Geometry check sheet. Reference: the model listing, model coordinates, mm. A direction names the side the tool comes from. Round coordinates to 2 decimals unless told otherwise and drop trailing zeros. One line per question, with ' | ' between items. Start each with the question number.
Q1. Gauge pin test, flat ends, axial feed: P1, Ø2.5, axis at y = 18.5, z = 26, coming from the -X side; P2, Ø3, axis at y = 230.5, z = 23.5, coming from the -X side; P3, Ø3, axis at y = 209.5, z = 26.5, coming from the -X side. Record the tip position at first contact, or that the pin passes through.
Q2. Tool access check on faces 1 (the face through (50, 20, 20)), 2 (the face through (-1, 15, 30)), 3 (the face through (-50, 21, 20)), 4 (the face through (59.14, 247.75, 37.97)). Record the directions out of +Z, -Z, +X, -X, +Y, -Y that give a thin tool (end or side, any length) a straight path to the whole face; none if there is none.
Q3. Material ranges on line 1 along X through (y, z) = (20, 23); line 2 along X through (y, z) = (155, 37); line 3 along X through (y, z) = (35, 16), recorded low to high.
Q4. Mould release check, pull along Y, two halves, no side actions. Record for faces 5 (the face through (4.78, 279.91, 19.76)), 6 (the face through (2, 157, 36)), 7 (the face through (40, 15, 20)): +Y half, -Y half, draft (parallel to the pull), parting line (faces both ways), or undercut.
```python
from build123d import *

# Parameters (mm, degrees)
SKETCH2_R           = 110
BOSS_EXTRUDE1_DEPTH = 40
SKETCH5_R           = 110
BOSS_EXTRUDE2_DEPTH = 36
FILLET1_R           = 3
SKETCH6_W           = 80
SKETCH6_H           = 20
CUT_EXTRUDE2_DEPTH  = 30
SKETCH7_W           = 70
SKETCH7_H           = 10
BOSS_EXTRUDE3_DEPTH = 30
SKETCH8_W           = 5
SKETCH8_H           = 30
BOSS_EXTRUDE4_DEPTH = 3


with BuildPart() as part:
    # Sketch2 → Boss-Extrude1 (new body)
    with BuildSketch(Plane.XY):
        with BuildLine():
            Line((-50, 0), (50, 0))
            Line((50, 0), (50, 40.435607626))
            ThreePointArc((50, 40.435607626), (0, 280), (-50, 40.435607626))
            Line((-50, 40.435607626), (-50, 0))
        make_face()
        with Locations((0, 155)):
            Circle(SKETCH2_R, mode=Mode.SUBTRACT)
    extrude(amount=BOSS_EXTRUDE1_DEPTH)

    # Sketch5 → Boss-Extrude2 (add)
    with BuildSketch(Plane(origin=(0, 0, 0), x_dir=(-1, 0, 0), z_dir=(0, 0, -1))):
        with Locations((0, 155)):
            Circle(SKETCH5_R)
    extrude(amount=-BOSS_EXTRUDE2_DEPTH)

    # Fillet1
    fillet1_edges = [part.edges().sort_by_distance(p)[0] for p in [
        (-50, 20.217803813, 40),
        (50, 20.217803813, 40),
        (-50, 20.217803813, 0),
        (0, 280, 0),
        (50, 20.217803813, 0),
        (0, 280, 40),
    ]]
    fillet(fillet1_edges, radius=FILLET1_R)

    # Sketch6 → Cut-Extrude2 (cut)
    with BuildSketch(Plane.XZ):
        with Locations((0, 20)):
            Rectangle(SKETCH6_W, SKETCH6_H)
    extrude(amount=-CUT_EXTRUDE2_DEPTH, mode=Mode.SUBTRACT)

    # Sketch7 → Boss-Extrude3 (add)
    with BuildSketch(Plane.XZ.offset(-30)):
        with Locations((0, 20)):
            Rectangle(SKETCH7_W, SKETCH7_H)
    extrude(amount=BOSS_EXTRUDE3_DEPTH)

    # Sketch8 → Boss-Extrude4 (add)
    with BuildSketch(Plane.XY.offset(25)):
        with Locations((-32.5, 15)):
            Rectangle(SKETCH8_W, SKETCH8_H)
        with Locations((-22.5, 15)):
            Rectangle(SKETCH8_W, SKETCH8_H)
        with Locations((-12.5, 15)):
            Rectangle(SKETCH8_W, SKETCH8_H)
        with Locations((-2.5, 15)):
            Rectangle(SKETCH8_W, SKETCH8_H)
        with Locations((7.5, 15)):
            Rectangle(SKETCH8_W, SKETCH8_H)
        with Locations((17.5, 15)):
            Rectangle(SKETCH8_W, SKETCH8_H)
        with Locations((27.5, 15)):
            Rectangle(SKETCH8_W, SKETCH8_H)
    boss_extrude4 = extrude(amount=BOSS_EXTRUDE4_DEPTH)

    # Mirror2: Boss-Extrude4 across plane
    add(boss_extrude4.mirror(Plane.XY.offset(21.007174775)))


solid = part.part
```
Determined:
1) P1: stops at x = -50 | P2: stops at x = -100.74 | P3: stops at x = -113.21
2) face 1: +Z, -Z, +X, -Y | face 2: -Y | face 3: +Z, -Z, -X, -Y | face 4: +Z
3) line 1: x = -50 to -40, -35 to 35, 40 to 50 | line 2: x = -125 to -110, 110 to 125 | line 3: x = -50 to 50
4) face 5: parting line | face 6: undercut | face 7: draft
